Part model, mm, in its own coordinate system. Face numbers are marked on the shaded views. A direction names the side the tool comes from. Coordinates: 2 decimals unless noted, no trailing zeros. Loops run counter-clockwise (first coordinate to the right, second up) from the corner with the lowest first, then second, coordinate; pieces in that order, holes last.
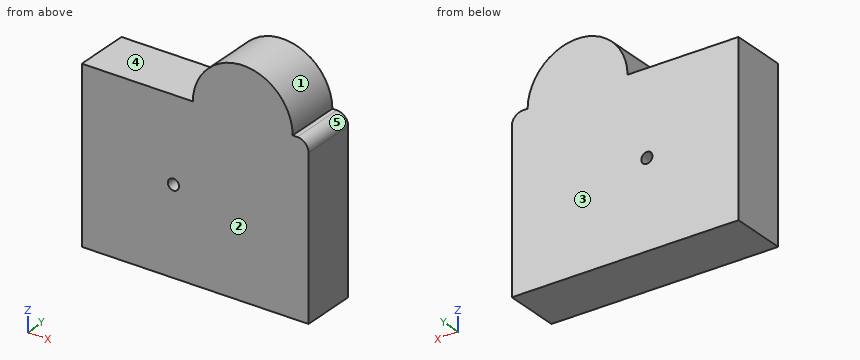
```python
from build123d import *

# Parameters (mm, degrees)
F0_W     = 101.6
F0_H     = 76.2
F1_DEPTH = 25
F2_R     = 5
F4_D     = 5
F5_R     = 22.404033
F6_DEPTH = 25


with BuildPart() as f1:
    # F0 (on Front) → F1 (new body)
    with BuildSketch(Plane.XZ):
        with Locations((9.736366, -0.770457)):
            Rectangle(F0_W, F0_H)
    extrude(amount=F1_DEPTH)

    # F2
    f2_edges = [f1.edges().sort_by_distance(p)[0] for p in [
        (60.536366, -12.5, 37.329543),
    ]]
    fillet(f2_edges, radius=F2_R)

    # F4 (through all)
    with Locations(Plane(origin=(0, 0, 0), x_dir=(-1, 0, 0), z_dir=(0, 1, 0))):
        with Locations((0, 0)):
            Hole(F4_D / 2)

    # F5 (on Front) → F6 (join)
    with BuildSketch(Plane.XZ):
        with Locations((31.058818, 37.010595)):
            Circle(F5_R)
    extrude(amount=F6_DEPTH)


solid = f1.part
```
Q1. Saw through at A-A (z = 0). List the corners of the cut face in (x, y), plus the area to 4 significant figures.
Q2. Tool access for the marked faces 4 and 5: list every direction of +Z, -Z, +X, -X, +Y, -Y with a clear straight run to the whole face (end or side of a thin tool).
Q3. Saw through at C-C (y = -9.25). List the corners of the cut face in (x, z), plus the area to 3 significant figures.
Q4. Drop flat-ended pins along their axis: P1, Ø3, axis at x = -5.5, y = -20, coming from the +Z side; P2, Ø8, axis at x = 0, z = 0, coming from the -Y side. Give the stop position or say it passes through.
Q5. Saw through at D-D (z = 52.5). List the corners of the cut face in (x, y).
Q6. Saw through at B-B (x = 0). List the corners of the cut face in (y, z), plus the area to 3 significant figures.
Q7. Probe line 1 (Z direction, x = 0, y = -10.75); line 2 (Z direction, x = 3.5, y = -8.5); line 3 (Z direction, x = 50, y = -23.5). List the from-to ranges inside material, lowest first.
Q8. Mould opens along Y. For the marked faces 1, 2 and 3 say: released by +Y, released by -Y, zero draft, split by the parting line, or undercut.
Checked values:
1. outline: (-41.06, -25) - (-2.5, -25) - (-2.5, 0) - (-41.06, 0) - close; (2.5, -25) - (60.54, -25) - (60.54, 0) - (2.5, 0) - close
1. area: 2,415 mm2
2. face 4: +Z, -X, +Y, -Y
2. face 5: +Z, +X, +Y, -Y
3. outline: (-41.06, -38.87) - (60.54, -38.87) - (60.54, 32.33) arc R5 ccw to (55.54, 37.33) - (53.46, 37.33) arc R22.4 ccw to (8.66, 37.33) - (-41.06, 37.33) - close; hole circle Ø5 at (0, 0)
3. area: 8,490 mm2
4. P1: stops at z = 37.33
4. P2: stops at y = -25
5. outline: (14.87, -25) - (47.25, -25) - (47.25, 0) - (14.87, 0) - close
6. outline: (-25, -38.87) - (0, -38.87) - (0, -2.5) - (-25, -2.5) - close; (-25, 2.5) - (0, 2.5) - (0, 37.33) - (-25, 37.33) - close
6. area: 1,780 mm2
7. line 1: z = -38.87 to -2.5, 2.5 to 37.33
7. line 2: z = -38.87 to 37.33
7. line 3: z = -38.87 to 48.98
8. face 1: zero draft
8. face 2: released by -Y
8. face 3: released by +Y
